Autodesk Inventor part; units mm, degrees
ref_plane "Start Plane" through (0, 0, 40) normal (0, 0, 1) x (1, 0, 0)
ref_plane "End Plane" through (0, 0, 210) normal (0, 0, 1) x (1, 0, 0)
ref_plane "Work Plane4" through (-6, 20, 40) normal (0, 0, -1) x (-1, 0, 0)
ref_plane "Start Plane" through (0, 0, 40) normal (0, 0, 1) x (1, 0, 0)
ref_plane "End Plane" through (0, 0, 210) normal (0, 0, 1) x (1, 0, 0)
sketch "Sketch" plane through (0, 0, 0) normal (0, 0, 1) x (1, 0, 0)
  line L0 (-10, -16) -> (-10, 16)
  line L1 (-6, 20) -> (6, 20)
  line L2 (10, 16) -> (10, -16)
  line L3 (6, -20) -> (-6, -20)
  arc A0 (-10, -16) -> (-6, -20) centre (-6, -16) ccw
  arc A1 (10, 16) -> (6, 20) centre (6, 16) ccw
  arc A2 (-6, 20) -> (-10, 16) centre (-6, 16) ccw
  arc A3 (6, -20) -> (10, -16) centre (6, -16) ccw
  arc A4 (-6, 18) -> (-8, 16) centre (-6, 16) ccw
  line L4 (-6, 18) -> (6, 18)
  arc A5 (8, 16) -> (6, 18) centre (6, 16) ccw
  line L5 (8, 16) -> (8, -16)
  arc A6 (6, -18) -> (8, -16) centre (6, -16) ccw
  line L6 (6, -18) -> (-6, -18)
  arc A7 (-8, -16) -> (-6, -18) centre (-6, -16) ccw
  line L7 (-8, -16) -> (-8, 16)
  line L8 (0, 29.1598) -> (0, -29.1598) construction
  line L9 (-15.1598, 0) -> (15.1598, 0) construction
  dimension "d7" = 4
  dimension "d9" = 20
  dimension "d11" = 40
  dimension "d12" = 2
  dimension "d15" = 10
  dimension "d16" = 20
extrude "Body" add sketch "Sketch" along normal up to surface (170 mm away) from surface at 40
sketch "Sketch3" plane through (0, 0, 0) normal (0, 0, 1) x (1, 0, 0)
  line L0 (0, 0) -> (10, 0)
ref_plane "Work Plane3" through (0, 0, 0) normal (0, -1, 0) x (1, 0, 0)
ref_plane "Work Plane4" through (-6, 20, 40) normal (0, 0, -1) x (-1, 0, 0)
split "Split1" plane through (-6, 20, 40) removes the side toward (0, 0, -1)
ref_plane "Work Plane5" through (-6, -580, 210) normal (0, 0, 1) x (1, 0, 0)
split "Split2" plane through (-6, -580, 210) removes the side toward (0, 0, 1)
sketch "Sketch4" plane through (0, 0, 0) normal (0, -1, 0) x (1, 0, 0)
  line L0 (-2, 40) -> (12, 40)
  line L1 (-2, 210) -> (12, 210)
  dimension "d18" = 170
equation "\"d7\" = G_IR"
equation "\"d9\" = G_W"
equation "\"d11\" = G_H"
equation "\"d12\" = G_T"
equation "\"d15\" = 0.5 * d9"
equation "\"d16\" = 0.5 * d11"
equation "\"d3\" = G_L"
equation "\"G_W\" = 20"
equation "\"G_H\" = 40"
equation "\"G_T\" = 2"
equation "\"G_IR\" = 4"
equation "\"G_L\" = d18"
properties part number "ISO 10799-2 - 40x20x2 - 170" material "Steel, Mild"
Build history of the part. All positions in model axes, mm. A direction names the side the tool comes from. Give positions to 0.01 mm unless a question says otherwise; leave off trailing zeros. Loops run counter-clockwise (first coordinate to the right, second up) from the corner with the lowest first, then second, coordinate; pieces in that order, holes last.
1) Two-plate mould, pull along X, no slides. Class faces 3 (the face through (0, 20, 124)), 4 (the face through (-8, 0, 124)), 5 (the face through (10, 0, 124)), 6 (the face through (8, 0, 124)): released by +X, released by -X, zero draft, split by the parting line, or undercut.
Values follow:
face 3: zero draft
face 4: undercut
face 5: released by +X
face 6: undercut
2) Band-saw the part on A-A on x = -0.5. List the corners of the cut face in (y, z), then the cut area to 3 significant figures.
Values follow:
outline: (-20, 40) - (-18, 40) - (-18, 210) - (-20, 210) - close; (18, 40) - (20, 40) - (20, 210) - (18, 210) - close
area: 680 mm2
3) Band-saw the part on B-B on y = 9. List the corners of the cut face in (x, z), then the cut area to 3 significant figures.
Values follow:
outline: (-10, 40) - (-8, 40) - (-8, 210) - (-10, 210) - close; (8, 40) - (10, 40) - (10, 210) - (8, 210) - close
area: 680 mm2
4) 3-axis set-ups, long thin cutter, end or side, ignore diameter. For faces 1 (the face through (-8.2, 0.1, 40)), 2 (the face through (0, -18, 124)): which of +Z, -Z, +X, -X, +Y, -Y reach the whole face in a straight line?
Values follow:
face 1: -Z, +X, -X, +Y, -Y
face 2: +Z, -Z
5) Band-saw the part on C-C on z = 143. List the corners of the cut face in (x, y), then the cut area to 3 significant figures.
Values follow:
outline: (-10, -16) arc R4 ccw to (-6, -20) - (6, -20) arc R4 ccw to (10, -16) - (10, 16) arc R4 ccw to (6, 20) - (-6, 20) arc R4 ccw to (-10, 16) - close; hole (-8, -16) arc R2 ccw to (-6, -18) - (6, -18) arc R2 ccw to (8, -16) - (8, 16) arc R2 ccw to (6, 18) - (-6, 18) arc R2 ccw to (-8, 16) - close
area: 214 mm2
6) Probe line 1 along X through (y, z) = (10, 62); line 2 along Y through (x, z) = (-5, 194.5); line 3 along Y through (x, z) = (7, 154). List the from-to ranges inside material, lowest first.
Values follow:
line 1: x = -10 to -8, 8 to 10
line 2: y = -20 to -18, 18 to 20
line 3: y = -19.87 to -17.73, 17.73 to 19.87
